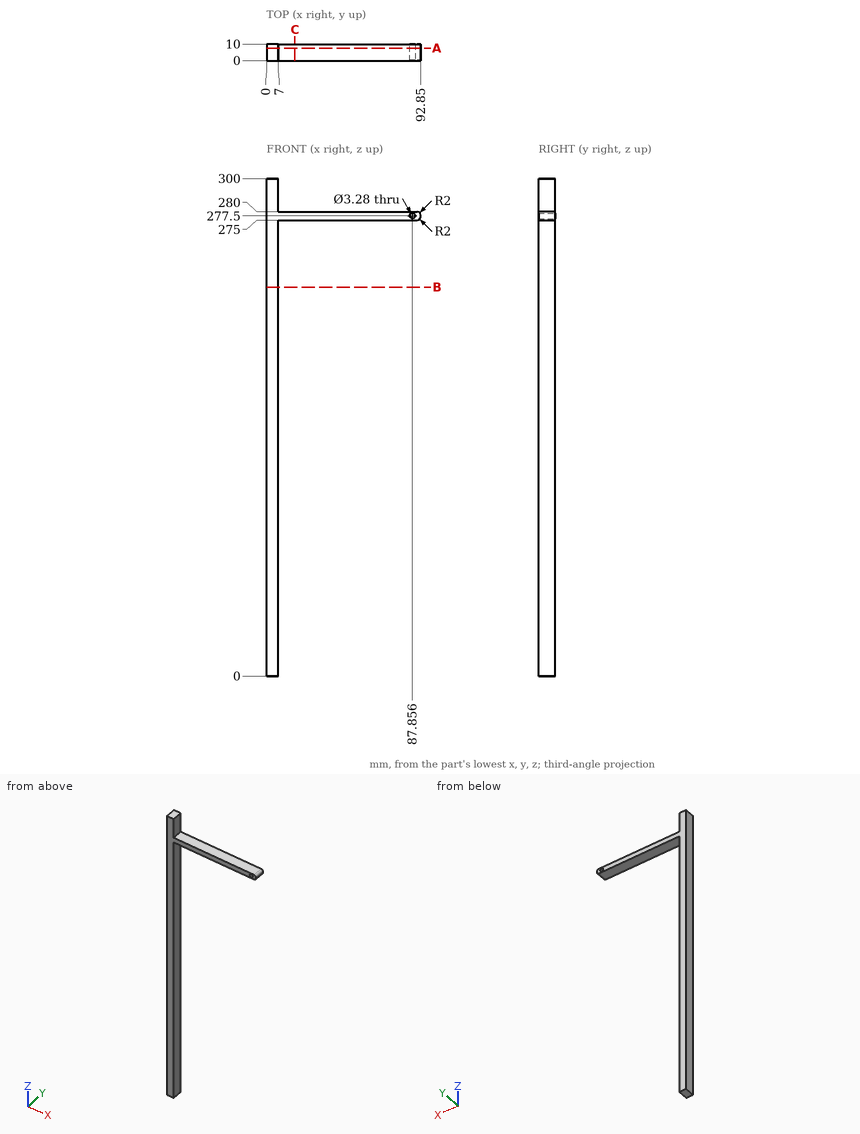
Answer from the drawing. Dimensions are ordinates in mm from the lowest x, y and z of the part. Coordinates: 2 decimals unless noted, no trailing zeros. Write each loop counter-clockwise with the first axis right and the second up, starting at its lowest first coordinate (ties: lowest second). Pieces come first, ordered by that corner, then holes. Notation, with made-up numbers: M 39.25,-28 L 46.25,-28 A26 cw 46.25,0 Z; hole C 9,43.25 d1. An arc over 180 degrees is marked long. Write item = value, one per line.
1. Straight lines are drawn through the part: line 1 (X direction, y = 4, z = 277.5); line 2 (Z direction, x = 52, y = 9); line 3 (X direction, y = 2.5, z = 53). For each, find the intervals that lie inside material, in ascending order. Write a range as from..to.
Solution:
line_1 = 0..86.22, 89.5..92.85
line_2 = 275..280
line_3 = 0..7
2. The part is cut by section A-A (y = 7.5). Determine the outline of the cut face in (x, z).
Solution:
outline = M 0,0 L 7,0 L 7,275 L 90.85,275 A2 ccw 92.85,277 L 92.85,278 A2 ccw 90.85,280 L 7,280 L 7,300 L 0,300 Z; hole C 87.86,277.5 d3.28
3. The part is cut by section B-B (z = 234.5). Determine the outline of the cut face in (x, y).
Solution:
outline = M 0,0 L 7,0 L 7,10 L 0,10 Z
4. The part is cut by section C-C (x = 17). Determine the outline of the cut face in (y, z).
Solution:
outline = M 0,275 L 10,275 L 10,280 L 0,280 Z
5. Flat-ended cylindrical pins translate along their axes: pin 1 (5 mm diameter, centred on y = 7.5, z = 165.5, fed in from +X); pin 2 (4 mm diameter, centred on x = 49, y = 3.5, fed in from +Z); pin 3 (3 mm diameter, centred on x = 58, y = 3, fed in from -Z). Find the tip coordinate at first contact, or state that the pin passes through.
Solution:
pin_1 = 7
pin_2 = 280
pin_3 = 275
